Answer from the drawing. Dimensions are ordinates in mm from the lowest x, y and z of the part. A direction names the side the tool comes from. Coordinates: 2 decimals unless noted, no trailing zeros. Loops run counter-clockwise (first coordinate to the right, second up) from the corner with the lowest first, then second, coordinate; pieces in that order, holes last. Notation, with made-up numbers: (35.5, 2) - (48.5, 2) arc R36 cw to (48.5, 41) - close; hole circle Ø10 at (9.5, 60). An arc over 180 degrees is marked (long way). Write each question's results on one line, items separated by ' | '. Start each with the question number.
1. A cutting plane is placed at C-C on x = 137. Determine the outline of the cut face in (y, z), then the cut area to 3 significant figures.
2. A cutting plane is placed at B-B on z = 55. Determine the outline of the cut face in (x, y) (1 decimal), then the cut area to 4 significant figures.
3. Which of the six approach directions +Z, -Z, +X, -X, +Y, -Y give full straight-line access (tool end or side, diameter ignored) to the marked faces 1, 2 and 3?
4. Determine the mould class of the marked faces 4, 5 and 6 for opening direction X: released by +X, released by -X, zero draft, split by the parting line, or undercut.
5. A cutting plane is placed at A-A on y = 30. State how many separate pieces and enclosed holes the cut face has, then the cut area to 3 significant figures.
6. Each of these flat-tipped pins is pushed along its axis until it touches: P1, Ø23.5, axis at y = 49, z = 43, coming from the -X side (1 decimal); P2, Ø5, axis at y = 36.5, z = 23, coming from the +X side; P3, Ø1.5, axis at x = 113, y = 15.5, coming from the +Z side; P4, Ø1.5, axis at x = 50.5, z = 29.5, coming from the -Y side. Where does it stop, or does it pass through?
7. Find the intervals of material crossed by line 1 along X through (y, z) = (16, 48.5) (1 decimal); line 2 along Z through (x, y) = (154, 39); line 3 along X through (y, z) = (32.5, 36.5) (1 decimal), in increasing order. Write a range as [from, to].
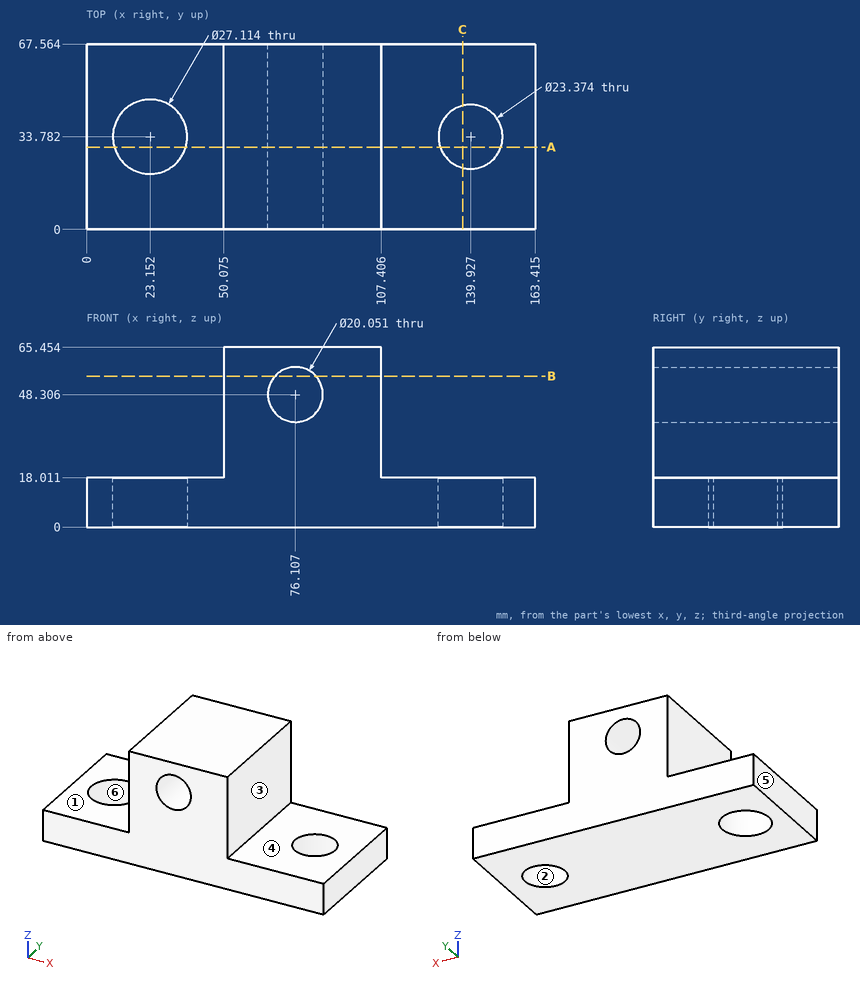
Values:
1) outline: (0, 0) - (22.47, 0) - (22.47, 18.01) - (0, 18.01) - close; (45.1, 0) - (67.56, 0) - (67.56, 18.01) - (45.1, 18.01) - close | area: 809 mm^2
2) outline: (50.1, 0) - (68.6, 0) - (68.6, 67.6) - (50.1, 67.6) - close; (83.6, 0) - (107.4, 0) - (107.4, 67.6) - (83.6, 67.6) - close | area: 2,865 mm^2
3) face 1: +Z, -X, +Y, -Y | face 2: +Z, -Z | face 3: +Z, +X, +Y, -Y
4) face 4: zero draft | face 5: released by -X | face 6: undercut
5) separate pieces: 3 | enclosed holes: 1 | area: 4,480 mm^2
6) P1: x = 50.1 | P2: x = 107.41 | P3: z = 18.01 | P4: y = 0
7) line 1: [50.1, 66.1], [86.1, 107.4] | line 2: [0, 18.01] | line 3: [50.1, 107.4]
